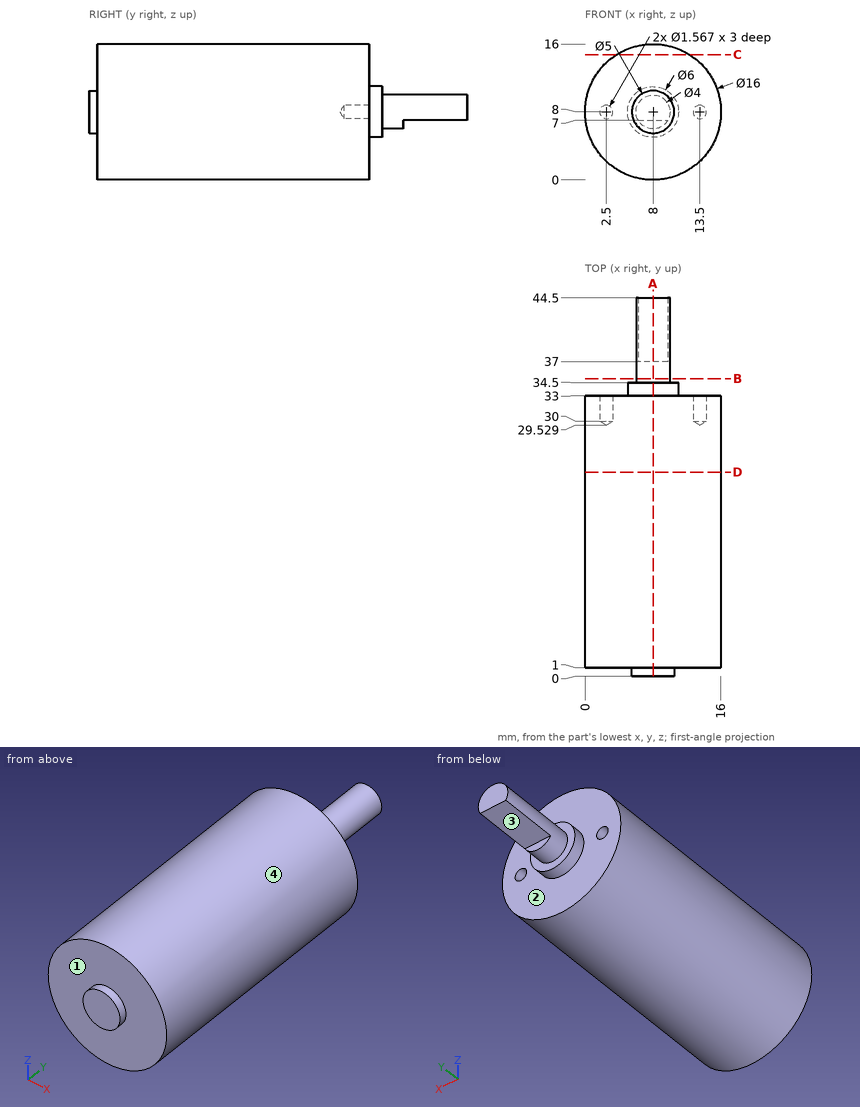
Print and shaded views of the part. All mm, measured from the part's lowest x, y and z. A direction names the side the tool comes from. Round coordinates to 2 decimals unless told otherwise and drop trailing zeros. Loops run counter-clockwise (first coordinate to the right, second up) from the corner with the lowest first, then second, coordinate; pieces in that order, holes last. Notation, with made-up numbers: (30, -3.5) -> (51, -3.5) arc R26 cw to (51, 18.5) -> close; hole circle Ø7 at (70, 78.5). An arc over 180 degrees is marked (long way). Use CSV: the item, a comma, the result in double quotes. Start each with the question number.
1) Cut at D-D, the plane y = 24. Write the cut outline in (x, z), plus the area to 3 significant figures.
2) Cut at A-A, the plane x = 8. Write the cut outline in (y, z).
3) Cut at C-C, the plane z = 14.75. Write the cut outline in (x, y), plus the area to 3 significant figures.
4) Cut at B-B, the plane y = 35. Write the cut outline in (x, z).
5) Drop flat-ended pins along their axis: P1, Ø4, axis at x = 9, y = 39, coming from the +Z side; P2, Ø1.8, axis at x = 2.5, z = 8, coming from the +Y side; P3, Ø5, axis at y = 31, z = 2.5, coming from the -X side. Give the stop position or say it passes through.
6) Which spindle directions (+Z, -Z, +X, -X, +Y, -Y) get a long thin tool onto all of the face, cutting with end or side? Do the marked faces 1, 2, 3 and 4. Say none if no direction does.
7) Wall check: L1, parallel to Z at x = 13.5, y = 31.6; L2, parallel to Y at x = 4, z = 7.75; L3, parallel to Y at x = 6.25, z = 6.25. Give the ranges that are in metal, low to high. Write a range as [from, to].
Determined:
1,outline,"circle Ø16 at (8, 8)"
1,area,"201 mm2"
2,outline,"(0, 5.5) -> (1, 5.5) -> (1, 0) -> (33, 0) -> (33, 5) -> (34.5, 5) -> (34.5, 6) -> (37, 6) -> (37, 7) -> (44.5, 7) -> (44.5, 10) -> (34.5, 10) -> (34.5, 11) -> (33, 11) -> (33, 16) -> (1, 16) -> (1, 10.5) -> (0, 10.5) -> close"
3,outline,"(3.71, 1) -> (12.29, 1) -> (12.29, 33) -> (3.71, 33) -> close"
3,area,"275 mm2"
4,outline,"circle Ø4 at (8, 8)"
5,P1,"stops at z = 10"
5,P2,"stops at y = 33"
5,P3,"stops at x = 0.58"
6,face 1,"-Y"
6,face 2,"+Y"
6,face 3,"-Z, +X, -X, +Y"
6,face 4,"+Y, -Y"
7,L1,"z = [2.19, 7.22], [8.78, 13.81]"
7,L2,"y = [1, 33]"
7,L3,"y = [0, 34.5]"
